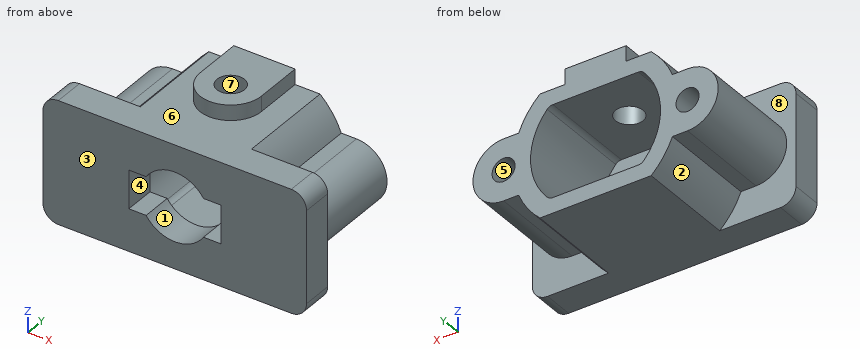
```python
from build123d import *

# Parameters (mm, degrees)
SKETCH_1_W               = 172
SKETCH_1_H               = 80
EXTRUDE_1_DEPTH          = 20
FILLET_1_R               = 10
SKETCH_2_R               = 7.5
EXTRUDE_2_DEPTH          = 65
CUT_EXTRUDE_1_DEPTH      = 65
EXTRUDE_3_DEPTH          = 10
CUT_EXTRUDE_2_DEPTH      = 10
CUT_EXTRUDE_2_DEPTH_BACK = 10
SKETCH_5_R               = 9
FILLET_2_R               = 5


with BuildPart() as part:
    # Sketch 1 → Extrude 1 (new body)
    with BuildSketch(Plane(origin=(0, 0, 0), x_dir=(1, 0, 0), z_dir=(0, 1, 0))):
        Rectangle(SKETCH_1_W, SKETCH_1_H)
        with BuildLine():
            Line((-30, -12.5), (-18.708286934, -12.5))
            ThreePointArc((-18.708286934, -12.5), (0, -22.5), (18.708286934, -12.5))
            Line((18.708286934, -12.5), (30, -12.5))
            Line((30, -12.5), (30, 12.5))
            Line((30, 12.5), (18.708286934, 12.5))
            ThreePointArc((18.708286934, 12.5), (0, 22.5), (-18.708286934, 12.5))
            Line((-18.708286934, 12.5), (-30, 12.5))
            Line((-30, 12.5), (-30, -12.5))
        make_face(mode=Mode.SUBTRACT)
    extrude(amount=EXTRUDE_1_DEPTH)

    # Fillet 1
    fillet_1_edges = [part.edges().sort_by_distance(p)[0] for p in [
        (86, 10, 40),
        (-86, 10, 40),
        (-86, 10, -40),
        (86, 10, -40),
    ]]
    fillet(fillet_1_edges, radius=FILLET_1_R)

    # Sketch 2 → Extrude 2 (add)
    with BuildSketch(Plane(origin=(0, 20, 0), x_dir=(1, 0, 0), z_dir=(0, 1, 0))):
        with BuildLine():
            Line((-36.276714294, 40), (36.276714294, 40))
            ThreePointArc((36.276714294, 40), (44.36006499, 30.792606809), (50.159744816, 20))
            Line((50.159744816, 20), (60, 20))
            ThreePointArc((60, 20), (80, 0), (60, -20))
            Line((60, -20), (50.159744816, -20))
            ThreePointArc((50.159744816, -20), (44.36006499, -30.792606809), (36.276714294, -40))
            Line((36.276714294, -40), (-36.276714294, -40))
            ThreePointArc((-36.276714294, -40), (-44.36006499, -30.792606809), (-50.159744816, -20))
            Line((-50.159744816, -20), (-60, -20))
            ThreePointArc((-60, -20), (-80, 0), (-60, 20))
            Line((-60, 20), (-50.159744816, 20))
            ThreePointArc((-50.159744816, 20), (-44.36006499, 30.792606809), (-36.276714294, 40))
        make_face()
        with Locations(Location((-60, 0, 0), (0, 0, 270))):
            Circle(SKETCH_2_R, mode=Mode.SUBTRACT)
        with Locations(Location((60, 0, 0), (0, 0, 270))):
            Circle(SKETCH_2_R, mode=Mode.SUBTRACT)
    extrude(amount=EXTRUDE_2_DEPTH)

    # Sketch 3 → Cut-Extrude 1 (cut)
    with BuildSketch(Plane(origin=(0, 20, 0), x_dir=(1, 0, 0), z_dir=(0, 1, 0))):
        with BuildLine():
            Line((-30, 30), (30, 30))
            ThreePointArc((30, 30), (42.426406871, 0), (30, -30))
            Line((30, -30), (-30, -30))
            ThreePointArc((-30, -30), (-42.426406871, 0), (-30, 30))
        make_face()
    extrude(amount=CUT_EXTRUDE_1_DEPTH, mode=Mode.SUBTRACT)

    # Sketch 4 → Extrude 3 (add)
    with BuildSketch(Plane.XY.offset(40)):
        with BuildLine():
            Line((-20, 53), (-20, 85))
            Line((-20, 85), (20, 85))
            Line((20, 85), (20, 53))
            ThreePointArc((20, 53), (0, 33), (-20, 53))
        make_face()
    extrude(amount=EXTRUDE_3_DEPTH)

    # Sketch 5 → Cut-Extrude 2 (cut, two sides: drawn at the far end of the back side and taken through both)
    with BuildSketch(Plane.XY.offset(40).offset(-CUT_EXTRUDE_2_DEPTH_BACK)):
        with Locations((0, 53)):
            Circle(SKETCH_5_R)
    extrude(amount=CUT_EXTRUDE_2_DEPTH + CUT_EXTRUDE_2_DEPTH_BACK, mode=Mode.SUBTRACT)

    # Fillet 2
    fillet_2_edges = [part.edges().sort_by_distance(p)[0] for p in [
        (30, 52.5, 30),
        (30, 52.5, -30),
        (-30, 52.5, -30),
        (-30, 52.5, 30),
    ]]
    fillet(fillet_2_edges, radius=FILLET_2_R)


solid = part.part
```
Can you work these out from the model? Positions are in its coordinate system, mm. Face numbers are marked on the shaded views. A direction names the side the tool comes from. Coordinates: 2 decimals unless noted, no trailing zeros. Order: outer loops, then holes, each group sorted by start corner. A loop starts at its lowest first (then second) coordinate and runs counter-clockwise, first axis right, second up.
1. I need wall thicknesses on line 1 (X direction, y = 56.5, z = 0); line 2 (Z direction, x = 8.5, y = 58); line 3 (X direction, y = 25, z = 3.5). Which ranges of each line are inside material? Lowest first, please.
2. For the marked faces 5, 6, 7 and 8, which set-ups out of +Z, -Z, +X, -X, +Y, -Y let a thin tool reach every point of the face, with its end or its side?
3. If we section it at D-D (y = 57): Give the number of separate pieces and of enclosed holes in the cut face, then the cut area to 3 significant figures.
4. If we section it at C-C (x = 0): Please give me the cut outline in (y, z), then the cut area to 3 significant figures.
5. I'm going to push flat-ended pins straight in: pin 1 (11 mm diameter, centred on y = 70.5, z = 43.5, fed in from +X); pin 2 (3 mm diameter, centred on x = 53, y = 37.5, fed in from +Z); pin 3 (11 mm diameter, centred on x = -56, y = 57.5, fed in from -Z). Where does each tip first touch, or does it pass through?
6. If we section it at B-B (z = 0): Please give me the cut outline in (x, y), then the cut area to 3 significant figures.
7. If we section it at A-A (y = 75): Please give me the cut outline in (x, z), then the cut area to 3 significant figures.
8. Thinking about a two-plate mould opening in Z: for the marked faces 1, 2, 3 and 4, which applies, +Z half, -Z half, draft (parallel to the pull), parting line (faces both ways), or undercut?
Entries:
1. line 1: x = -80 to -67.5, -52.5 to -42.43, 42.43 to 52.5, 67.5 to 80
1. line 2: z = -40 to -30, 30 to 50
1. line 3: x = -79.69 to -66.63, -53.37 to -42.28, 42.28 to 53.37, 66.63 to 79.69
2. face 5: +Y
2. face 6: +Z, -Y
2. face 7: +Z
2. face 8: -X, +Y
3. separate pieces: 1
3. enclosed holes: 2
3. area: 4,700 mm2
4. outline: (0, -40) - (85, -40) - (85, -30) - (20, -30) - (20, -22.5) - (0, -22.5) - close; (0, 22.5) - (20, 22.5) - (20, 30) - (44, 30) - (44, 50) - (33, 50) - (33, 40) - (0, 40) - close; (62, 30) - (85, 30) - (85, 50) - (62, 50) - close
4. area: 2,160 mm2
5. pin 1: stops at x = 38.37
5. pin 2: stops at z = 20
5. pin 3: stops at z = -20
6. outline: (-86, 0) - (-30, 0) - (-30, 20) - (-42.43, 20) - (-42.43, 85) - (-52.5, 85) - (-52.5, 20) - (-67.5, 20) - (-67.5, 85) - (-80, 85) - (-80, 20) - (-86, 20) - close; (30, 0) - (86, 0) - (86, 20) - (80, 20) - (80, 85) - (67.5, 85) - (67.5, 20) - (52.5, 20) - (52.5, 85) - (42.43, 85) - (42.43, 20) - (30, 20) - close
6. area: 5,170 mm2
7. outline: (-60, -20) - (-50.16, -20) arc R54 ccw to (-36.28, -40) - (36.28, -40) arc R54 ccw to (50.16, -20) - (60, -20) arc R20 ccw to (60, 20) - (50.16, 20) arc R54 ccw to (36.28, 40) - (20, 40) - (20, 50) - (-20, 50) - (-20, 40) - (-36.28, 40) arc R54 ccw to (-50.16, 20) - (-60, 20) arc R20 ccw to start; hole circle Ø15 at (-60, 0); hole (-31.57, -28.34) arc R5 ccw to (-27.85, -30) - (27.85, -30) arc R5 ccw to (31.57, -28.34) arc R42.43 ccw to (31.57, 28.34) arc R5 ccw to (27.85, 30) - (-27.85, 30) arc R5 ccw to (-31.57, 28.34) arc R42.43 ccw to start; hole circle Ø15 at (60, 0)
7. area: 5,030 mm2
8. face 1: undercut
8. face 2: -Z half
8. face 3: draft
8. face 4: undercut
